Model file for the job. Use its own axes, mm. Round coordinates to 2 decimals unless told otherwise and drop trailing zeros. Order: outer loops, then holes, each group sorted by start corner. A loop starts at its lowest first (then second) coordinate and runs counter-clockwise, first axis right, second up. Notation, with made-up numbers: (71, -27.5) -> (95, -27.5) arc R24 cw to (95, 1.5) -> close; hole circle Ø10 at (-11, 30.25). An arc over 180 degrees is marked (long way). Answer as CSV lines item,"result".
Autodesk Inventor part; units mm, degrees
ref_plane "Work Plane1" through (-3.4, -3.4, -4.5) normal (0, 0, -1) x (0, 1, 0)
ref_plane "YZ Plane" through (0, 0, 0) normal (1, 0, 0) x (0, 1, 0)
ref_plane "XZ Plane" through (0, 0, 0) normal (0, 1, 0) x (-1, 0, 0)
sketch "Sketch1" plane through (0, 0, 0) normal (0, 0, 1) x (1, 0, 0)
  line L0 (-2.3998, 1.6282) -> (-2.4042, 2.4042)
  arc A0 (-2.3998, 1.6282) -> (-2.8482, 0.5456) centre (0, 0) ccw
  line L1 (-3.4, 0) -> (-2.8482, 0.5456)
  line L2 (-2.8482, -0.5456) -> (-3.4, 0)
  arc A1 (-2.8482, -0.5456) -> (-2.3998, -1.6282) centre (0, 0) ccw
  line L3 (-2.4042, -2.4042) -> (-2.3998, -1.6282)
  line L4 (-1.6282, -2.3998) -> (-2.4042, -2.4042)
  arc A2 (-1.6282, -2.3998) -> (-0.5456, -2.8482) centre (0, 0) ccw
  line L5 (0, -3.4) -> (-0.5456, -2.8482)
  line L6 (0.5456, -2.8482) -> (0, -3.4)
  arc A3 (0.5456, -2.8482) -> (1.6282, -2.3998) centre (0, 0) ccw
  line L7 (2.4042, -2.4042) -> (1.6282, -2.3998)
  line L8 (2.3998, -1.6282) -> (2.4042, -2.4042)
  arc A4 (2.3998, -1.6282) -> (2.8482, -0.5456) centre (0, 0) ccw
  line L9 (3.4, 0) -> (2.8482, -0.5456)
  line L10 (2.8482, 0.5456) -> (3.4, 0)
  arc A5 (2.8482, 0.5456) -> (2.3998, 1.6282) centre (0, 0) ccw
  line L11 (2.4042, 2.4042) -> (2.3998, 1.6282)
  line L12 (1.6282, 2.3998) -> (2.4042, 2.4042)
  arc A6 (1.6282, 2.3998) -> (0.5456, 2.8482) centre (0, 0) ccw
  line L13 (0, 3.4) -> (0.5456, 2.8482)
  line L14 (-0.5456, 2.8482) -> (0, 3.4)
  arc A7 (-0.5456, 2.8482) -> (-1.6282, 2.3998) centre (0, 0) ccw
  line L15 (-2.4042, 2.4042) -> (-1.6282, 2.3998)
  circle A8 centre (0, 0) radius 1
  circle A9 centre (0, 0) radius 2.9
  circle A10 centre (0, 0) radius 1.1
  line L16 (-12.5394, 7.938) -> (-12.4815, -3.7618)
  line L17 (-12.4815, -3.7618) -> (12.5182, -3.6381)
  line L18 (12.5182, -3.6381) -> (12.4603, 8.0618)
  line L19 (12.4603, 8.0618) -> (-12.5394, 7.938)
  circle A11 centre (8.485, 3.042) radius 3
  circle A12 centre (-8.5147, 2.9579) radius 3
  line L20 (0, 0) -> (0.0183, -3.7)
  line L21 (0.0183, -3.7) -> (0.0243, -4.8999)
  circle A13 centre (0, 0) radius 4.9
  point P0 (0, 0)
  dimension "d0" = 1.2
ref_plane "Work Plane1" through (-3.4, -3.4, -4.5) normal (0, 0, -1) x (0, 1, 0)
extrude "Extrusion1" add sketch "Sketch1" against normal up to surface (4.5 mm away) contours L17 A13 | L17 A13 L21 | L21 A13 L17
properties part number "oponka"
Q1. Saw through at A-A (z = -2). Write the cut outline in (x, y).
Checks:
outline,"circle Ø9.8 at (0, 0); hole (-3.4, 0) -> (-2.85, -0.55) arc R2.9 ccw to (-2.4, -1.63) -> (-2.4, -2.4) -> (-1.63, -2.4) arc R2.9 ccw to (-0.55, -2.85) -> (0, -3.4) -> (0.55, -2.85) arc R2.9 ccw to (1.63, -2.4) -> (2.4, -2.4) -> (2.4, -1.63) arc R2.9 ccw to (2.85, -0.55) -> (3.4, 0) -> (2.85, 0.55) arc R2.9 ccw to (2.4, 1.63) -> (2.4, 2.4) -> (1.63, 2.4) arc R2.9 ccw to (0.55, 2.85) -> (0, 3.4) -> (-0.55, 2.85) arc R2.9 ccw to (-1.63, 2.4) -> (-2.4, 2.4) -> (-2.4, 1.63) arc R2.9 ccw to (-2.85, 0.55) -> close"
Q2. Flat gauge pins, fed straight in: pin 1 (1 mm diameter, centred on y = 1, z = -2.5, fed in from +X); pin 2 (4 mm diameter, centred on x = -1.5, y = -2.5, fed in from +Z). Where does each tip first touch, or does it go through?
Checks:
pin 1,"x = 4.87"
pin 2,"z = 0"
Q3. Saw through at B-B (y = 1). Write the cut outline in (x, z), plus the area to 3 significant figures.
Checks:
outline,"(-4.8, -4.5) -> (-2.72, -4.5) -> (-2.72, 0) -> (-4.8, 0) -> close; (2.72, -4.5) -> (4.8, -4.5) -> (4.8, 0) -> (2.72, 0) -> close"
area,"18.7 mm²"
Q4. Saw through at D-D (x = -4). Write the cut outline in (y, z).
Checks:
outline,"(-2.83, -4.5) -> (2.83, -4.5) -> (2.83, 0) -> (-2.83, 0) -> close"
Q5. Wall check: L1, parallel to X at y = 0.5, z = -2.5; L2, parallel to X at y = -3.25, z = -4.05; L3, parallel to Y at x = 2, z = -1.35. Give the ranges that are in metal, low to high. Write a range as [from, to].
Checks:
L1,"[-4.87, -2.89], [2.89, 4.87]"
L2,"[-3.67, -0.15], [0.15, 3.67]"
L3,"[-4.47, -2.4], [2.4, 4.47]"
Q6. Saw through at C-C (x = 0.75). Write the cut outline in (y, z).
Checks:
outline,"(-4.84, -4.5) -> (-2.8, -4.5) -> (-2.8, 0) -> (-4.84, 0) -> close; (2.8, -4.5) -> (4.84, -4.5) -> (4.84, 0) -> (2.8, 0) -> close"
